Work out the finished part from the listing and answer in its coordinate system (mm). A direction names the side the tool comes from. Give positions to 0.01 mm unless a question says otherwise; leave off trailing zeros. Loops run counter-clockwise (first coordinate to the right, second up) from the corner with the lowest first, then second, coordinate; pieces in that order, holes last.
```python
from build123d import *

# Parameters (mm, degrees)
CUT_EXTRUDE1_REACH = 157.644
SKETCH3_R          = 15.443252693


with BuildPart() as part:
    # Sketch2 → Revolve1 (revolve)
    with BuildSketch(Plane(origin=(0, 0, 0), x_dir=(0, 0, -1), z_dir=(1, 0, 0))):
        Polygon((-10, 76.5), (-10, 73.5), (-9, 72.5), (-5, 72.5), (-5, -76.5), (-4, -77.5), (0, -77.5), (0, 77.5), (-9, 77.5), align=None)
    revolve(axis=Axis((0, 23.60486684, 0), (0, -1, 0)))

    # Cut-Extrude1: up to this face of the body (flat: up to its plane)
    cut_extrude1_end = Plane(part.part.faces().sort_by_distance((0, 72.5, -8.745441559))[0])
    # Sketch3 → Cut-Extrude1 (cut, up to the picked face)
    with BuildSketch(Plane(origin=(0, 77.5, 0), x_dir=(1, 0, 0), z_dir=(0, 1, 0)), mode=Mode.PRIVATE) as cut_extrude1_sk1:
        Circle(SKETCH3_R)
        Polygon((0, -9.814954576), (8.5, -4.907477288), (8.5, 4.907477288), (0, 9.814954576), (-8.5, 4.907477288), (-8.5, -4.907477288), align=None, mode=Mode.SUBTRACT)
    cut_extrude1_tool1 = split(extrude(cut_extrude1_sk1.sketch, amount=-CUT_EXTRUDE1_REACH, mode=Mode.PRIVATE), bisect_by=cut_extrude1_end, keep=Keep.BOTH, mode=Mode.PRIVATE)
    add(cut_extrude1_tool1.solids().sort_by(Axis((-15.006452, 77.5, 0), (0, -1, 0)))[0], mode=Mode.SUBTRACT)


solid = part.part
```
Q1. Which of the six approach directions +Z, -Z, +X, -X, +Y, -Y give full straight-line access (tool end or side, diameter ignored) to faces 1 (the face through (4.88, -3.04, -1.08)), 2 (the face through (-4.309, 75.035, 7.327))?
Q2. Consider line 1 along Z through (x, y) = (3, -24); line 2 along X through (y, z) = (-5, -1); line 3 along Y through (x, z) = (5.75, 1). Determine where each line is inside the solid, lowest interval first.
Q3. Section A-A on z = 0 is taken. Give the vertices of the cut face in (x, y), plus the area to 3 significant figures.
Q4. Section B-B on y = 38 is taken. Give the vertices of the cut face in (x, z).
Q5. Given pin 1 (8 mm diameter, centred on x = -6, y = 37, fed in from +Z); pin 2 (4 mm diameter, centred on y = -6.5, z = 4, fed in from +X); pin 3 (5 mm diameter, centred on x = -5.5, y = -57.5, fed in from +Z), each flat-ended and moving along its own axis, determine where each tip first touches the part or whether it passes through.
Check result:
1. face 1: -Y
1. face 2: +Z, -X, +Y, -Y
2. line 1: z = -4 to 4
2. line 2: x = -4.9 to 4.9
2. line 3: y = 72.5 to 77.5
3. outline: (-8.5, 72.5) - (-5, 72.5) - (-5, -76.5) - (-4, -77.5) - (4, -77.5) - (5, -76.5) - (5, 72.5) - (8.5, 72.5) - (8.5, 77.5) - (-8.5, 77.5) - close
3. area: 1,580 mm2
4. outline: circle Ø10 at (0, 0)
5. pin 1: stops at z = 4.58
5. pin 2: stops at x = 4.58
5. pin 3: stops at z = 4
